Part model, mm, in its own coordinate system. Face numbers are marked on the shaded views. A direction names the side the tool comes from. Coordinates: 2 decimals unless noted, no trailing zeros. Write each loop counter-clockwise with the first axis right and the second up, starting at its lowest first coordinate (ties: lowest second). Pieces come first, ordered by that corner, then holes. Notation, with made-up numbers: (59.25, 87) -> (71.25, 87) arc R24 ccw to (71.25, 98) -> close; hole circle Ø5 at (17.5, 4). An arc over 180 degrees is marked (long way). Write item = value, one per line. Start each with the question number.
Q1. Pin check, flat tips, straight feed: P1, Ø8, axis at y = 7.5, z = 53, coming from the -X side; P2, Ø5, axis at y = 10, z = 66, coming from the -X side; P3, Ø5.5, axis at x = 27, y = 9, coming from the +Z side. Stop position of each tip, or through.
Q2. Band-saw the part on B-B, the plane y = 10. Give the number of separate pieces and of enclosed holes in the cut face, plus the area to 3 significant figures.
Q3. Tool access for the marked faces 1 and 2: list every direction of +Z, -Z, +X, -X, +Y, -Y with a clear straight run to the whole face (end or side of a thin tool).
Q4. Band-saw the part on A-A, the plane z = 24. List the corners of the cut face in (x, y).
Q5. Probe line 1 (Z direction, x = 43.8, y = 10); line 2 (X direction, y = 11.5, z = 26.5); line 3 (Z direction, x = 14.5, y = 10). List the from-to ranges inside material, lowest first.
Q6. Pull direction X, two halves, no side cores. Call the marked faces 3, 4 and 5: released by +X, released by -X, zero draft, split by the parting line, or undercut.
Q7. Band-saw the part on D-D, the plane y = 18.5. List the corners of the cut face in (x, z).
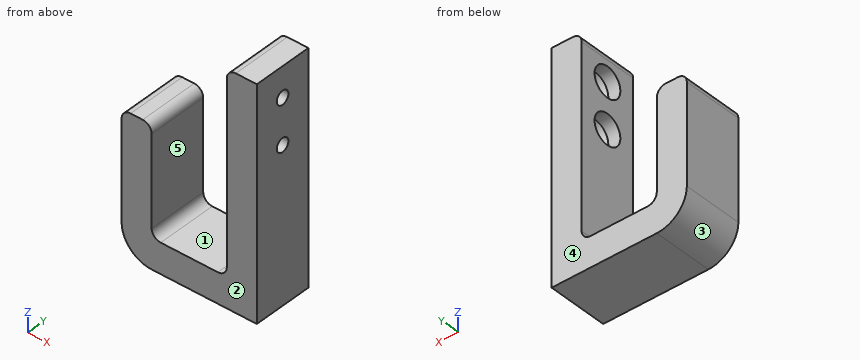
Autodesk Fusion 360 part; units mm, degrees
sketch "Sketch1" plane through (0, 0, 0) normal (0, 1, 0) x (1, 0, 0)
  line L0 (10, -46) -> (10, -10)
  line L1 (10, -10) -> (35, -10)
  line L2 (35, -10) -> (35, -76)
  line L3 (35, -76) -> (45, -76)
  line L4 (45, -76) -> (45, 0)
  line L5 (45, 0) -> (0, 0)
  line L6 (0, 0) -> (0, -46)
  line L7 (0, -46) -> (10, -46)
  dimension "d1" = 36
  dimension "d2" = 25
  dimension "d3" = 10
  dimension "d4" = 10
  dimension "d5" = 10
  dimension "d6" = 30
extrude "Extrude1" add sketch "Sketch1" along normal blind 20
sketch "Sketch2" plane through (35, 0, 0) normal (-1, 0, 0) x (0, -1, 0)
  line L0 (0, 10) -> (0, 76)
  line L1 (0, 76) -> (-20, 76)
  line L2 (-20, 76) -> (-20, 10)
  line L3 (-20, 10) -> (0, 10)
  circle A0 centre (-10, 66) radius 5
  circle A1 centre (-10, 51) radius 5
  line L4 (-20, 76) -> (-10, 66) construction
  line L5 (-10, 66) -> (0, 76) construction
  line L6 (-10, 66) -> (-10, 51) construction
  circle A2 centre (-10, 66) radius 2.25
  circle A3 centre (-10, 51) radius 2.25
  dimension "d9" = 10
  dimension "d11" = 15
  dimension "d12" = 10
  dimension "d13" = 10
  dimension "d14" = 4.5
  dimension "d15" = 4.5
extrude "Extrude2" cut sketch "Sketch2" against normal up to surface (10 mm away) contours A2 | A3
extrude "Extrude3" cut sketch "Sketch2" against normal blind 4 contours A0 | A1
chamfer "Chamfer1" distance 2.75 angle 45 2 edges at (39, 12.0977, 65.1864) (39, 12.0977, 50.1864)
fillet "Fillet2" radius 3 5 edges at (35, 10, 76) (35, 10, 10) (10, 10, 10) (10, 10, 46) (0, 10, 46)
fillet "Fillet2" radius 10 1 edges at (0, 10, 0)
equation "d13 = d9"
equation "d15 = d14"
Ans:
q1.P1 = 35
q1.P2 = 41.5
q1.P3 = 10
q2.separate_pieces = 3
q2.enclosed_holes = 0
q2.area = 1,300 mm2
q3.face_1 = +Z, +Y, -Y
q3.face_2 = +Z, -Z, +X, -X, -Y
q4.outline = (0, 0) -> (10, 0) -> (10, 20) -> (0, 20) -> close; (35, 0) -> (45, 0) -> (45, 20) -> (35, 20) -> close
q5.line_1 = 0 to 48.75, 53.25 to 63.75, 68.25 to 76
q5.line_2 = 0 to 10, 35 to 45
q5.line_3 = 0 to 10
q6.face_3 = released by -X
q6.face_4 = zero draft
q6.face_5 = undercut
q7.outline = (0, 10) arc R10 ccw to (10, 0) -> (45, 0) -> (45, 76) -> (38, 76) arc R3 ccw to (35, 73) -> (35, 13) arc R3 cw to (32, 10) -> (13, 10) arc R3 cw to (10, 13) -> (10, 43) arc R3 ccw to (7, 46) -> (3, 46) arc R3 ccw to (0, 43) -> close
